Source: CAD feature listing. Evaluate the final solid. Frame: model axes, mm. Face numbers are marked on the shaded views. A direction names the side the tool comes from. Round coordinates to 2 decimals unless told otherwise and drop trailing zeros. Order: outer loops, then holes, each group sorted by start corner. A loop starts at its lowest first (then second) coordinate and runs counter-clockwise, first axis right, second up. Notation, with made-up numbers: (-40, 62.5) -> (-15, 62.5) arc R33 cw to (-15, 100.5) -> close; hole circle Ø4 at (84, 26.5). An arc over 180 degrees is marked (long way). One line per item, written item: value. Start each with the question number.
1) Ray query, L1, parallel to Y at x = 108, z = -2; L2, parallel to X at y = -319.5, z = -59; L3, parallel to X at y = -209, z = -23.5. Return the intervals inside material, ascending.
2) Section A-A (x = 0). Return the cut outline in (y, z), and give its area (3 significant figures).
3) Reachability of the marked faces 1 and 2 from +Z, -Z, +X, -X, +Y, -Y: full face, straight path, thin tool, end or side. Return the list, or none.
4) Section D-D (z = -107). Return the cut outline in (x, y).
5) Section B-B (z = 0). Return the cut outline in (x, y), and give its area (3 significant figures).
6) Pin query (flat end, axial travel): P1, Ø6, axis at x = 57.5, y = -245.5, coming from the -Z side; P2, Ø4, axis at y = -74.5, z = 74, coming from the +X side; P3, Ø11, axis at x = 84.85, z = -84.85, coming from the +Y side; P4, Ø12, axis at x = -79, y = -166.5, coming from the +Z side. Return the tip coordinate at first contact, or that it passes through.
7) Section C-C (y = -182.5). Return the cut outline in (x, z).
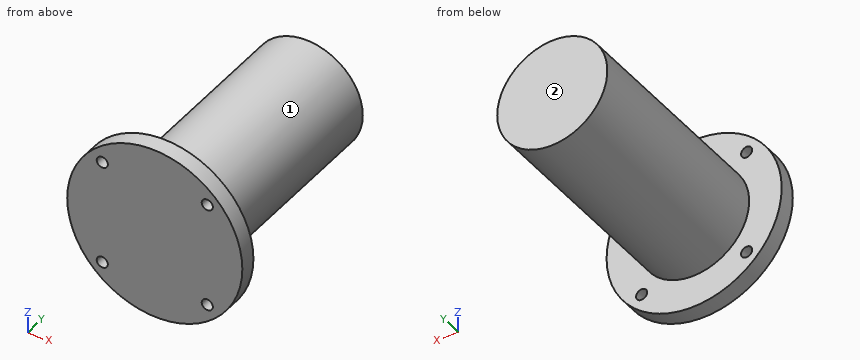
```python
from build123d import *

# Parameters (mm, degrees)
F0_R     = 89
F1_DEPTH = 345
F2_R     = 141.5
F3_DEPTH = 27
F4_R     = 9
F5_DEPTH = 372.001


with BuildPart() as f1:
    # F0 (on Front) → F1 (new body)
    with BuildSketch(Plane.XZ):
        Circle(F0_R)
    extrude(amount=F1_DEPTH)

    # F2 (on face) → F3 (join)
    with BuildSketch(Plane.XZ.offset(345)):
        Circle(F2_R)
    extrude(amount=F3_DEPTH)

    # F4 (on face) → F5 (cut, through all)
    with BuildSketch(Plane.XZ.offset(372)):
        with Locations((-84.852814, 84.852814)):
            Circle(F4_R)
        with Locations((-84.852814, -84.852814)):
            Circle(F4_R)
        with Locations((84.852814, -84.852814)):
            Circle(F4_R)
        with Locations((84.852814, 84.852814)):
            Circle(F4_R)
    extrude(amount=-F5_DEPTH, mode=Mode.SUBTRACT)


solid = f1.part
```
Findings:
1. L1: -372 to -345
1. L2: -66.63 to 66.63
1. L3: -85.84 to 85.84
2. outline: (-372, -141.5) -> (-345, -141.5) -> (-345, -89) -> (0, -89) -> (0, 89) -> (-345, 89) -> (-345, 141.5) -> (-372, 141.5) -> close
2. area: 69,100 mm2
3. face 1: +Y
3. face 2: +Z, -Z, +X, -X, +Y
4. outline: (-92.59, -372) -> (92.59, -372) -> (92.59, -345) -> (-92.59, -345) -> close
5. outline: (-141.5, -372) -> (141.5, -372) -> (141.5, -345) -> (89, -345) -> (89, 0) -> (-89, 0) -> (-89, -345) -> (-141.5, -345) -> close
5. area: 69,100 mm2
6. P1: z = -70.36
6. P2: x = 52.32
6. P3: through
6. P4: z = 50.91
7. outline: circle Ø178 at (0, 0)
